from build123d import *

# Parameters (mm, degrees)
F0_R     = 1.5
F1_DEPTH = 2


with BuildPart() as f1:
    # F0 (on Top) → F1 (new body)
    with BuildSketch(Plane.XY):
        Polygon((23.795815, 21.350004), (23.795815, 16.350004), (33.795815, 16.350004), (33.795815, 21.350004), (33.795815, 26.350004), (28.795815, 26.350004), (28.795815, 21.350004), align=None)
        with Locations((27.545815, 18.850004)):
            Circle(F0_R, mode=Mode.SUBTRACT)
        with Locations((31.295815, 18.850004)):
            Circle(F0_R, mode=Mode.SUBTRACT)
        with Locations((31.295815, 22.600004)):
            Circle(F0_R, mode=Mode.SUBTRACT)
    extrude(amount=F1_DEPTH)


solid = f1.part
Could you check a few things on this model? Use its own coordinates, in mm. A direction names the side the tool comes from. Coordinates: 2 decimals unless noted, no trailing zeros. Order: outer loops, then holes, each group sorted by start corner. A loop starts at its lowest first (then second) coordinate and runs counter-clockwise, first axis right, second up. Notation, with made-up numbers: (42.25, 88.25) - (49.25, 88.25) arc R4 ccw to (49.25, 95.25) - close; hole circle Ø5 at (8.5, 25). An arc over 180 degrees is marked (long way). Answer in a Markdown table with one row per item. Add a question column.
(1) If we section it at D-D, the plane y = 23.25: Please give me the cut outline in (x, z), then the cut area to 3 significant figures.
(2) If we section it at A-A, the plane z = 1.35: Please give me the cut outline in (x, y).
(3) If we mould it in two halves opening along X, with no side actions, what happens to faces 1 (the face through (30, 20, 2)), 2 (the face through (26.047, 18.916, 0.986)), 3 (the face through (33.796, 21, 1))? For each: released by +X, released by -X, zero draft, split by the parting line, or undercut.
(4) If we section it at B-B, the plane x = 30: Please give me the cut outline in (y, z), then the cut area to 3 significant figures.
(5) On a 3-axis mill with a long thin cutter (end or side, diameter ignored), from which of +Z, -Z, +X, -X, +Y, -Y can I reach the whole of each face in a straight line? I mean faces 4 (the face through (29.797, 18.916, 0.986)), 5 (the face through (26, 21.35, 1)). Say none if no direction works.
(6) I need wall thicknesses on L1, parallel to X at y = 18.75, z = 0.35; L2, parallel to X at y = 19.5, z = 1.7; L3, parallel to Y at x = 25.5, z = 0.45. Which ranges of each line are inside material? Lowest first, please.
(7) Will these pins go through, and if not, where does the flat tip stop? pin 1 (2.5 mm diameter, centred on x = 31.3, y = 18.85, fed in from -Z); pin 2 (0.6 mm diameter, centred on x = 27, z = 0.5, fed in from +Y).
(8) If we section it at C-C, the plane y = 17.5: Please give me the cut outline in (x, z), then the cut area to 3 significant figures.
Results are:
| question | item | result |
|---|---|---|
| 1 | outline | (28.8, 0) - (29.94, 0) - (29.94, 2) - (28.8, 2) - close; (32.65, 0) - (33.8, 0) - (33.8, 2) - (32.65, 2) - close |
| 1 | area | 4.59 mm2 |
| 2 | outline | (23.8, 16.35) - (33.8, 16.35) - (33.8, 26.35) - (28.8, 26.35) - (28.8, 21.35) - (23.8, 21.35) - close; hole circle Ø3 at (27.55, 18.85); hole circle Ø3 at (31.3, 18.85); hole circle Ø3 at (31.3, 22.6) |
| 3 | face 1 | zero draft |
| 3 | face 2 | undercut |
| 3 | face 3 | released by +X |
| 4 | outline | (16.35, 0) - (18.09, 0) - (18.09, 2) - (16.35, 2) - close; (19.61, 0) - (21.84, 0) - (21.84, 2) - (19.61, 2) - close; (23.36, 0) - (26.35, 0) - (26.35, 2) - (23.36, 2) - close |
| 4 | area | 14.0 mm2 |
| 5 | face 4 | +Z, -Z |
| 5 | face 5 | +Z, -Z, -X, +Y |
| 6 | L1 | x = 23.8 to 26.05, 29.04 to 29.8, 32.79 to 33.8 |
| 6 | L2 | x = 23.8 to 26.19, 28.9 to 29.94, 32.65 to 33.8 |
| 6 | L3 | y = 16.35 to 21.35 |
| 7 | pin 1 | passes through |
| 7 | pin 2 | stops at y = 21.35 |
| 8 | outline | (23.8, 0) - (26.89, 0) - (26.89, 2) - (23.8, 2) - close; (28.2, 0) - (30.64, 0) - (30.64, 2) - (28.2, 2) - close; (31.95, 0) - (33.8, 0) - (33.8, 2) - (31.95, 2) - close |
| 8 | area | 14.8 mm2 |
